Read the model definition and answer for the solid it produces. Units are mm, in the model's axes. Face numbers are marked on the shaded views. A direction names the side the tool comes from. Coordinates: 2 decimals unless noted, no trailing zeros. Write each loop counter-clockwise with the first axis right and the second up, starting at its lowest first coordinate (ties: lowest second). Pieces come first, ordered by that corner, then holes. Notation, with made-up numbers: M 79,44.5 L 88,44.5 A29 cw 88,71.5 Z; hole C -27,6.25 d7. An arc over 180 degrees is marked long. Write item = value, one per line.
from build123d import *

# Parameters (mm, degrees)
SKETCH1_R           = 60
BOSS_EXTRUDE1_DEPTH = 440
SKETCH2_R           = 41
BOSS_EXTRUDE2_DEPTH = 90
SKETCH3_R           = 41
BOSS_EXTRUDE3_DEPTH = 90
SKETCH4_R           = 39
BOSS_EXTRUDE4_DEPTH = 103.75
SKETCH5_R           = 39
BOSS_EXTRUDE5_DEPTH = 103.75
SKETCH6_R           = 34
BOSS_EXTRUDE6_DEPTH = 6.25
SKETCH7_R           = 34
BOSS_EXTRUDE7_DEPTH = 6.25
SKETCH8_R           = 3.75
CUT_EXTRUDE1_DEPTH  = 840


with BuildPart() as part:
    # Sketch1 → Boss-Extrude1 (new body)
    with BuildSketch(Plane.XY):
        Circle(SKETCH1_R)
    extrude(amount=BOSS_EXTRUDE1_DEPTH)

    # Sketch2 → Boss-Extrude2 (add)
    with BuildSketch(Plane(origin=(0, 0, 0), x_dir=(-1, 0, 0), z_dir=(0, 0, -1))):
        Circle(SKETCH2_R)
    extrude(amount=BOSS_EXTRUDE2_DEPTH)

    # Sketch3 → Boss-Extrude3 (add)
    with BuildSketch(Plane.XY.offset(440)):
        Circle(SKETCH3_R)
    extrude(amount=BOSS_EXTRUDE3_DEPTH)

    # Sketch4 → Boss-Extrude4 (add)
    with BuildSketch(Plane.XY.offset(530)):
        Circle(SKETCH4_R)
    extrude(amount=BOSS_EXTRUDE4_DEPTH)

    # Sketch5 → Boss-Extrude5 (add)
    with BuildSketch(Plane(origin=(0, 0, -90), x_dir=(-1, 0, 0), z_dir=(0, 0, -1))):
        Circle(SKETCH5_R)
    extrude(amount=BOSS_EXTRUDE5_DEPTH)

    # Sketch6 → Boss-Extrude6 (add)
    with BuildSketch(Plane(origin=(0, 0, -193.75), x_dir=(-1, 0, 0), z_dir=(0, 0, -1))):
        Circle(SKETCH6_R)
    extrude(amount=BOSS_EXTRUDE6_DEPTH)

    # Sketch7 → Boss-Extrude7 (add)
    with BuildSketch(Plane.XY.offset(633.75)):
        Circle(SKETCH7_R)
    extrude(amount=BOSS_EXTRUDE7_DEPTH)

    # Sketch8 → Cut-Extrude1 (cut)
    with BuildSketch(Plane.XY.offset(640)):
        Circle(SKETCH8_R)
    extrude(amount=-CUT_EXTRUDE1_DEPTH, mode=Mode.SUBTRACT)


solid = part.part
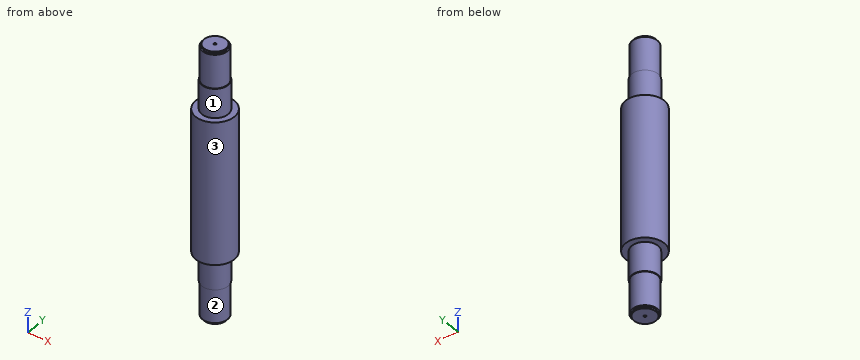
Item 1: Find section D-D (z = 370.5). Determine the outline of the cut face in (x, y).
Worked answers:
outline = C 0,0 d120; hole C 0,0 d7.5
Item 2: Consider line 1 along Y through (x, z) = (0, 469); line 2 along Y through (x, z) = (0, 157); line 3 along Z through (x, y) = (-12, -32). Determine where each line is inside the solid, lowest interval first. Write a range as from..to.
Worked answers:
line_1 = -41..-3.75, 3.75..41
line_2 = -60..-3.75, 3.75..60
line_3 = -193.75..633.75
Item 3: Find section B-B (y = -12.5). Determine the outline of the cut face in (x, z).
Worked answers:
outline = M -58.68,0 L -39.05,0 L -39.05,-90 L -36.94,-90 L -36.94,-193.75 L -31.62,-193.75 L -31.62,-200 L 31.62,-200 L 31.62,-193.75 L 36.94,-193.75 L 36.94,-90 L 39.05,-90 L 39.05,0 L 58.68,0 L 58.68,440 L 39.05,440 L 39.05,530 L 36.94,530 L 36.94,633.75 L 31.62,633.75 L 31.62,640 L -31.62,640 L -31.62,633.75 L -36.94,633.75 L -36.94,530 L -39.05,530 L -39.05,440 L -58.68,440 Z
Item 4: Which of the six approach directions +Z, -Z, +X, -X, +Y, -Y give full straight-line access (tool end or side, diameter ignored) to the marked faces 1, 2 and 3?
Worked answers:
face_1 = +Z
face_2 = -Z
face_3 = +Z, -Z
Item 5: Flat-ended cylindrical pins translate along their axes: pin 1 (6 mm diameter, centred on x = -39.5, y = -39, fed in from -Z); pin 2 (10 mm diameter, centred on x = -25.5, z = 225, fed in from +Y); pin 3 (3 mm diameter, centred on x = 17.5, y = -31, fed in from +Z); pin 4 (8.5 mm diameter, centred on x = 0, y = 0, fed in from +Z). Find the tip coordinate at first contact, or state that the pin passes through.
Worked answers:
pin_1 = 0
pin_2 = 56.39
pin_3 = 633.75
pin_4 = 640
Item 6: Find section C-C (x = 26.5). Determine the outline of the cut face in (y, z), and give its area (3 significant figures).
Worked answers:
outline = M -53.83,0 L -31.28,0 L -31.28,-90 L -28.61,-90 L -28.61,-193.75 L -21.3,-193.75 L -21.3,-200 L 21.3,-200 L 21.3,-193.75 L 28.61,-193.75 L 28.61,-90 L 31.28,-90 L 31.28,0 L 53.83,0 L 53.83,440 L 31.28,440 L 31.28,530 L 28.61,530 L 28.61,633.75 L 21.3,633.75 L 21.3,640 L -21.3,640 L -21.3,633.75 L -28.61,633.75 L -28.61,530 L -31.28,530 L -31.28,440 L -53.83,440 Z
area = 71,000 mm²
Item 7: Find section A-A (z = 477.5). Determine the outline of the cut face in (x, y), and give its area (3 significant figures).
Worked answers:
outline = C 0,0 d82; hole C 0,0 d7.5
area = 5,240 mm²
